Input: part model. Units: mm. Frame: model coordinates. Face numbers are marked on the shaded views. A direction names the side the tool comes from. Give positions to 0.01 mm unless a question says otherwise; leave off trailing zeros. Loops run counter-clockwise (first coordinate to the right, second up) from the corner with the lowest first, then second, coordinate; pieces in that order, holes last. Notation, with made-up numbers: M 31.25,2.5 L 58.25,2.5 A17 ccw 58.25,23.5 Z; hole C 71.5,-8.5 d8. An arc over 180 degrees is marked long. Answer as a JSON object with one key per item and string values. Group by question number.
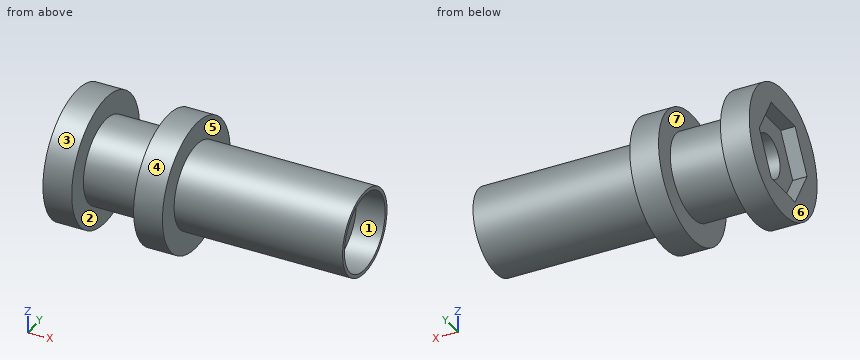
```python
from build123d import *

# Parameters (mm, degrees)
SKETCH1_R               = 2.95
BOSS_EXTRUDE1_DEPTH     = 18
SKETCH2_R               = 2.7
CUT_EXTRUDE1_DEPTH      = 2
CUT_EXTRUDE2_DEPTH      = 17.534962957
CUT_EXTRUDE2_DEPTH_BACK = 17.534962957
SKETCH3_R               = 1.5
SKETCH4_R               = 4.5
BOSS_EXTRUDE2_DEPTH     = 2
BOSS_EXTRUDE3_START     = -6.3
SKETCH4_3_R             = 4.5
BOSS_EXTRUDE3_DEPTH     = 2
CUT_EXTRUDE3_DEPTH      = 21.988091862
CUT_EXTRUDE3_DEPTH_BACK = 21.988091862
SKETCH5_R               = 1.5
CUT_EXTRUDE4_DEPTH      = 21.988091862
CUT_EXTRUDE4_DEPTH_BACK = 1


with BuildPart() as part:
    # Sketch1 → Boss-Extrude1 (new body)
    with BuildSketch(Plane(origin=(0, 0, 0), x_dir=(0, 0, -1), z_dir=(1, 0, 0))):
        Circle(SKETCH1_R)
    extrude(amount=BOSS_EXTRUDE1_DEPTH)

    # Sketch2 → Cut-Extrude1 (cut)
    with BuildSketch(Plane(origin=(18, 0, 0), x_dir=(0, 0, -1), z_dir=(1, 0, 0))):
        Circle(SKETCH2_R)
    extrude(amount=-CUT_EXTRUDE1_DEPTH, mode=Mode.SUBTRACT)

    # Sketch3 → Cut-Extrude2 (cut, two sides: drawn at the far end of the back side and taken through both)
    with BuildSketch(Plane(origin=(16, 0, 0), x_dir=(0, 0, -1), z_dir=(1, 0, 0)).offset(-CUT_EXTRUDE2_DEPTH_BACK)):
        Circle(SKETCH3_R)
    extrude(amount=CUT_EXTRUDE2_DEPTH + CUT_EXTRUDE2_DEPTH_BACK, mode=Mode.SUBTRACT)

    # Sketch4 → Boss-Extrude2 (add)
    with BuildSketch(Plane.ZY):
        Circle(SKETCH4_R)
    extrude(amount=BOSS_EXTRUDE2_DEPTH)

    # Sketch4<3> → Boss-Extrude3 (add)
    with BuildSketch(Plane.ZY.offset(BOSS_EXTRUDE3_START)):
        Circle(SKETCH4_3_R)
    extrude(amount=BOSS_EXTRUDE3_DEPTH)

    # Sketch5 → Cut-Extrude3 (cut, two sides: drawn at the far end of the back side and taken through both)
    with BuildSketch(Plane.ZY.offset(2).offset(-CUT_EXTRUDE3_DEPTH_BACK)):
        with Locations(Location((0, 0, 0), (0, 0, 180))):
            Circle(SKETCH5_R)
    extrude(amount=CUT_EXTRUDE3_DEPTH + CUT_EXTRUDE3_DEPTH_BACK, mode=Mode.SUBTRACT)

    # Sketch6 → Cut-Extrude4 (cut, two sides: drawn at the far end of the back side and taken through both)
    with BuildSketch(Plane.ZY.offset(2).offset(-CUT_EXTRUDE4_DEPTH_BACK)):
        Polygon((2.75, -1.58771324), (2.75, 1.58771324), (0, 3.175426481), (-2.75, 1.58771324), (-2.75, -1.58771324), (0, -3.175426481), align=None)
    extrude(amount=CUT_EXTRUDE4_DEPTH + CUT_EXTRUDE4_DEPTH_BACK, mode=Mode.SUBTRACT)


solid = part.part
```
1. Section B-B (y = 0). Output: boundary loops of the cut face in (x, z), then the cut area to 3 significant figures.
2. Mould query, pull axis X, two halves, no side actions, for the marked faces 4, 5, 6 and 7. Classes: pulls with the +X half, pulls with the -X half, needs draft (parallel to the pull), parting line crosses it, or undercut.
3. Material intervals for L1, parallel to X at y = 2.75, z = 1.25; L2, parallel to Y at x = 17.6, z = 0; L3, parallel to Z at x = 4, y = 0, sorted ascending.
4. Section C-C (x = 15.25). Output: boundary loops of the cut face in (y, z), then the cut area to 3 significant figures.
5. Section D-D (z = 2.25). Output: boundary loops of the cut face in (x, y), then the cut area to 3 significant figures.
6. Section A-A (z = -1.25). Output: boundary loops of the cut face in (x, y).
7. Reachability of the marked faces 1, 2 and 3 from +Z, -Z, +X, -X, +Y, -Y: full face, straight path, thin tool, end or side. Return the list, or none.
8. First-contact query: P1, Ø1, axis at x = 8.5, y = 1.5, coming from the -Z side; P2, Ø3.5, axis at y = 0, z = 0, coming from the -X side; P3, Ø2, axis at x = 1.5, y = -1.5, coming from the +Z side; P4, Ø1.6, axis at y = 0, z = 0, coming from the -X side. Flat tips, straight axial feed; report the tip coordinate or a pass-through.
Geometry results:
{
 "1": {"outline": "M -2,-4.5 L 0,-4.5 L 0,-2.95 L 4.3,-2.95 L 4.3,-4.5 L 6.3,-4.5 L 6.3,-2.95 L 18,-2.95 L 18,-2.7 L 16,-2.7 L 16,-1.5 L -1,-1.5 L -1,-2.75 L -2,-2.75 Z; M -2,2.75 L -1,2.75 L -1,1.5 L 16,1.5 L 16,2.7 L 18,2.7 L 18,2.95 L 6.3,2.95 L 6.3,4.5 L 4.3,4.5 L 4.3,2.95 L 0,2.95 L 0,4.5 L -2,4.5 Z", "area": "63.1 mm2"},
 "2": {"face 4": "needs draft", "face 5": "pulls with the +X half", "face 6": "pulls with the -X half", "face 7": "undercut"},
 "3": {"L1": "-2 to 0, 4.3 to 6.3", "L2": "-2.95 to -2.7, 2.7 to 2.95", "L3": "-2.95 to -1.5, 1.5 to 2.95"},
 "4": {"outline": "C 0,0 d5.9; hole C 0,0 d3", "area": "20.3 mm2"},
 "5": {"outline": "M -2,-3.9 L 0,-3.9 L 0,-1.91 L 4.3,-1.91 L 4.3,-3.9 L 6.3,-3.9 L 6.3,-1.91 L 18,-1.91 L 18,-1.49 L 16,-1.49 L 16,1.49 L 18,1.49 L 18,1.91 L 6.3,1.91 L 6.3,3.9 L 4.3,3.9 L 4.3,1.91 L 0,1.91 L 0,3.9 L -2,3.9 L -2,1.88 L -1,1.88 L -1,-1.88 L -2,-1.88 Z", "area": "82.5 mm2"},
 "6": {"outline": "M -2,-4.32 L 0,-4.32 L 0,-2.67 L 4.3,-2.67 L 4.3,-4.32 L 6.3,-4.32 L 6.3,-2.67 L 18,-2.67 L 18,-2.39 L 16,-2.39 L 16,-0.83 L -1,-0.83 L -1,-2.45 L -2,-2.45 Z; M -2,2.45 L -1,2.45 L -1,0.83 L 16,0.83 L 16,2.39 L 18,2.39 L 18,2.67 L 6.3,2.67 L 6.3,4.32 L 4.3,4.32 L 4.3,2.67 L 0,2.67 L 0,4.32 L -2,4.32 Z"},
 "7": {"face 1": "+X", "face 2": "none", "face 3": "+X, -X"},
 "8": {"P1": "z = -2.78", "P2": "x = -1", "P3": "z = 2.91", "P4": "through"}
}
